The figure shows three views and two pictorial views of one solid part (mm, origin at its lowest corner). Answer the questions. A direction names the side the tool comes from. Coordinates: 2 decimals unless noted, no trailing zeros. Order: outer loops, then holes, each group sorted by start corner. A loop starts at its lowest first (then second) coordinate and runs counter-clockwise, first axis right, second up. Notation, with made-up numbers: M -39.75,-21 L 13.25,-21 A3 cw 13.25,-16 Z; hole C 34,40.25 d3. An arc over 180 degrees is marked long. Write item = value, one per line. Start each with the question number.
Q1. Find section B-B on y = 16. Give the vertices of the cut face in (x, z), and give its area (3 significant figures).
Q2. Straight lines are drawn through the part: line 1 along Y through (x, z) = (33, 2.75); line 2 along X through (y, z) = (32.5, 2); line 3 along Y through (x, z) = (44.5, 6.5). For each, find the intervals that lie inside material, in ascending order.
Q3. Find section D-D on x = 19.5. Give the vertices of the cut face in (y, z), and give its area (3 significant figures).
Q4. Find section A-A on z = 1.5. Give the vertices of the cut face in (x, y), and give its area (3 significant figures).
Q5. Each of these flat-tipped pins is pushed along its axis until it touches: P1, Ø1.2, axis at y = 2.5, z = 6, coming from the -X side; P2, Ø1.2, axis at y = 3, z = 7.5, coming from the +X side. Where does it stop, or does it pass through?
Q6. Determine the mould class of the marked faces 1, 2 and 3 for opening direction Z: released by +Z, released by -Z, zero draft, split by the parting line, or undercut.
Q7. A tool of negligible diameter and unlimited length cuts with its end or side. For the marked faces 4, 5 and 6, from which of +Z, -Z, +X, -X, +Y, -Y can it reach the whole face along a straight path? Write none if from no direction.
Q8. Find section C-C on x = 44. Give the vertices of the cut face in (y, z).
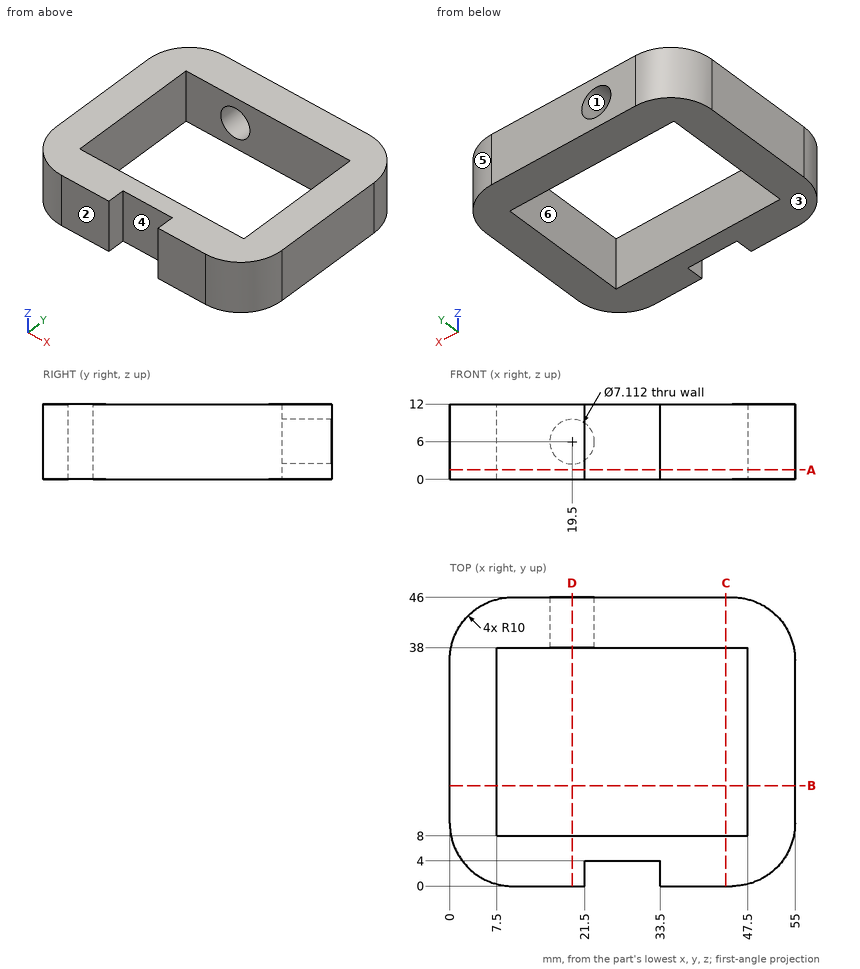
Findings below:
q1.outline = M 0,0 L 7.5,0 L 7.5,12 L 0,12 Z; M 47.5,0 L 55,0 L 55,12 L 47.5,12 Z
q1.area = 180 mm^2
q2.line_1 = 4 to 8, 38 to 46
q2.line_2 = 0 to 7.5, 47.5 to 55
q2.line_3 = 0 to 8, 38 to 46
q3.outline = M 0,0 L 8,0 L 8,12 L 0,12 Z; M 38,0 L 46,0 L 46,2.44 L 38,2.44 Z; M 38,9.56 L 46,9.56 L 46,12 L 38,12 Z
q3.area = 135 mm^2
q4.outline = M 0,10 A10 ccw 10,0 L 21.5,0 L 21.5,4 L 33.5,4 L 33.5,0 L 45,0 A10 ccw 55,10 L 55,36 A10 ccw 45,46 L 10,46 A10 ccw 0,36 Z; hole M 7.5,8 L 47.5,8 L 47.5,38 L 7.5,38 Z
q4.area = 1,200 mm^2
q5.P1 = 2.76
q5.P2 = 52.68
q6.face_1 = undercut
q6.face_2 = zero draft
q6.face_3 = released by -Z
q7.face_4 = +Z, -Z, -Y
q7.face_5 = +Z, -Z, +X, +Y
q7.face_6 = +Z, -Z
q8.outline = M 0,0 L 8,0 L 8,12 L 0,12 Z; M 38,0 L 46,0 L 46,12 L 38,12 Z
